Part model, mm, in its own coordinate system. A direction names the side the tool comes from. Give positions to 0.01 mm unless a question says otherwise; leave off trailing zeros. Write each loop counter-clockwise with the first axis right and the second up, starting at its lowest first coordinate (ties: lowest second). Pieces come first, ordered by that corner, then holes. Notation, with made-up numbers: M -22.5,9 L 5.5,9 A14 ccw 5.5,33 Z; hole C 7,-29.75 d6. An arc over 180 degrees is marked long. Use CSV: the item, a comma, the result in double quotes. Start each with the question number.
Item 1: Drill centre lines: line 1 (Y direction, x = 69.5, z = 66); line 2 (X direction, y = 493.5, z = 238.5); line 3 (Y direction, x = 245, z = 279.5). Where is each one in solid material? Low to high. Write a range as [from, to].
Item 2: Mould opens along X. For faces 1 (the flat face through (0, 9, 148)), 2 (the flat face through (256, 9, 300)), 3 (the flat face through (257, 512, 157)) say: released by +X, released by -X, zero draft, split by the parting line, or undercut.
Item 3: Cut at C-C (x = 168.5). List the corners of the cut face in (y, z).
Item 4: Cut at B-B (y = 459). List the corners of the cut face in (x, z).
Item 5: Cut at A-A (z = 100.5). List the corners of the cut face in (x, y), then the cut area to 3 significant figures.
Item 6: Which spindle directions (+Z, -Z, +X, -X, +Y, -Y) get a long thin tool onto all of the face, cutting with end or side? Do faces 4 (the flat face through (26, 273, 282)), 5 (the flat face through (502, 270, 148)), 6 (the flat face through (257, 36, 157)). Say none if no direction does.
Item 7: Pin check, flat tips, straight feed: pin 1 (12 mm diameter, centred on y = 143.5, z = 91.5, fed in from -X); pin 2 (1 mm diameter, centred on x = 188.5, y = 313.5, fed in from +Z); pin 3 (2 mm diameter, centred on y = 232, z = 193.5, fed in from +X). Stop position of each tip, or through.
from build123d import *

# Parameters (mm, degrees)
F0_W     = 520
F0_H     = 300
F0_W_2   = 484
F0_H_2   = 264
F1_DEPTH = 18
F2_DEPTH = 530
F3_W     = 448
F3_H     = 476
F4_DEPTH = 253
F6_DEPTH = 545


with BuildPart() as f1:
    # F0 (on Front) → F1 (new body)
    with BuildSketch(Plane.XZ):
        with Locations((260, 150)):
            Rectangle(F0_W, F0_H)
        with Locations((260, 150)):
            Rectangle(F0_W_2, F0_H_2, mode=Mode.SUBTRACT)
    extrude(amount=-F1_DEPTH)

    # F0 (on Front) → F2 (join)
    with BuildSketch(Plane.XZ):
        with Locations((260, 150)):
            Rectangle(F0_W_2, F0_H_2)
    extrude(amount=-F2_DEPTH)

    # F3 (on face) → F4 (cut)
    with BuildSketch(Plane.XY.offset(282)):
        with Locations((260, 274)):
            Rectangle(F3_W, F3_H)
    extrude(amount=-F4_DEPTH, mode=Mode.SUBTRACT)

    # F5 (on face) → F6 (cut)
    with BuildSketch(Plane(origin=(0, 0, 0), x_dir=(0, -1, 0), z_dir=(-1, 0, 0))):
        with BuildLine():
            Line((-5, 260), (0, 260))
            Line((0, 260), (0, 289))
            ThreePointArc((0, 289), (-5, 294), (-10, 289))
            Line((-10, 289), (-10, 265))
            ThreePointArc((-10, 265), (-8.535534, 261.464466), (-5, 260))
        make_face()
    extrude(amount=-F6_DEPTH, mode=Mode.SUBTRACT)


solid = f1.part
Worked answers:
1,line 1,"y = [0, 36], [512, 530]"
1,line 2,"x = [18, 36], [484, 502]"
1,line 3,"y = [10, 36], [512, 530]"
2,face 1,"released by -X"
2,face 2,"zero draft"
2,face 3,"undercut"
3,outline,"M 0,0 L 18,0 L 18,18 L 530,18 L 530,282 L 512,282 L 512,29 L 36,29 L 36,282 L 18,282 L 18,300 L 0,300 L 0,289 A5 cw 10,289 L 10,265 A5 cw 5,260 L 0,260 Z"
4,outline,"M 18,18 L 502,18 L 502,282 L 484,282 L 484,29 L 36,29 L 36,282 L 18,282 Z"
5,outline,"M 0,0 L 520,0 L 520,18 L 502,18 L 502,530 L 18,530 L 18,18 L 0,18 Z; hole M 36,36 L 484,36 L 484,512 L 36,512 Z"
5,area,"43,900 mm^2"
6,face 4,"+Z, +X, -X, +Y"
6,face 5,"+Z, -Z, +X, +Y"
6,face 6,"+Z"
7,pin 1,"stops at x = 18"
7,pin 2,"stops at z = 29"
7,pin 3,"stops at x = 502"
